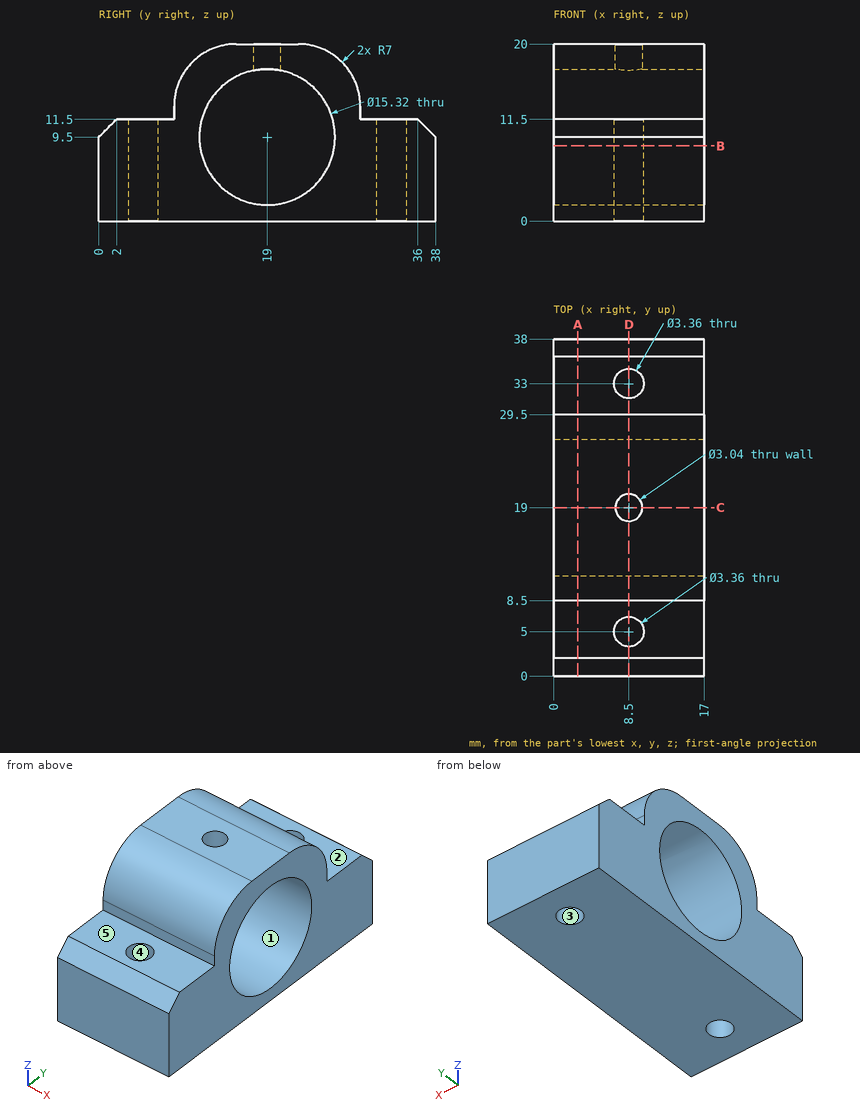
Design review of the part shown in the three views and the two pictorial views. Dimensions are in mm from the part's minimum x, y and z. A direction names the side the tool comes from. Round coordinates to 2 decimals unless told otherwise and drop trailing zeros. Loops run counter-clockwise (first coordinate to the right, second up) from the corner with the lowest first, then second, coordinate; pieces in that order, holes last. Notation, with made-up numbers: M 13.25,-14 L 66.25,-14 A24 ccw 66.25,25 Z; hole C 10.25,24 d11. An arc over 180 degrees is marked long. Write item = value, one per line.
Item 1: Take a section at A-A on x = 2.75. Write out the cut boundary in (y, z).
Return value:
outline = M 0,0 L 38,0 L 38,9.5 L 36,11.5 L 29.5,11.5 L 29.5,13 A7 ccw 22.5,20 L 15.5,20 A7 ccw 8.5,13 L 8.5,11.5 L 2,11.5 L 0,9.5 Z; hole C 19,9.5 d15.32
Item 2: For line 1 (Z direction, x = 13, y = 19); line 2 (X direction, y = 19, z = 17.6); line 3 (X direction, y = 33, z = 8), list the stretches that pass through material, from the lowest coordinate up. Write a range as [from, to].
Return value:
line_1 = [0, 1.84], [17.16, 20]
line_2 = [0, 6.98], [10.02, 17]
line_3 = [0, 6.82], [10.18, 17]
Item 3: Insertion check: P1, Ø2, axis at x = 4.5, z = 11, coming from the -Y side; P2, Ø1.5, axis at y = 21.5, z = 4, coming from the -X side; P3, Ø2, axis at x = 3.5, y = 25, coming from the +Z side; P4, Ø1.2, axis at x = 9.5, z = 12, coming from the +Y side. Each pin has a flat end and moves straight along its axis. Give the tip position at first contact, or say it passes through.
Return value:
P1 = 0.5
P2 = through
P3 = 19.84
P4 = 36.1
Item 4: Machinability: for the marked faces 4 and 5, which of the approach directions +Z, -Z, +X, -X, +Y, -Y give a long, thin tool a straight path to every point of the face, cutting with its end or side? Answer none if there is none.
Return value:
face_4 = +Z, -Z
face_5 = +Z, +X, -X, -Y
Item 5: Take a section at C-C on y = 19. Write out the cut boundary in (x, z).
Return value:
outline = M 0,0 L 17,0 L 17,1.84 L 0,1.84 Z; M 0,17.16 L 6.98,17.16 L 6.98,20 L 0,20 Z; M 10.02,17.16 L 17,17.16 L 17,20 L 10.02,20 Z
Item 6: The part is to be moulded in two halves that separate along Z. For the marked faces 1, 2 and 3, say which applies: released by +Z, released by -Z, zero draft, split by the parting line, or undercut.
Return value:
face_1 = undercut
face_2 = released by +Z
face_3 = zero draft
Item 7: Take a section at D-D on x = 8.5. Write out the cut boundary in (y, z).
Return value:
outline = M 0,0 L 3.32,0 L 3.32,11.5 L 2,11.5 L 0,9.5 Z; M 6.68,0 L 31.32,0 L 31.32,11.5 L 29.5,11.5 L 29.5,13 A7 ccw 22.5,20 L 20.52,20 L 20.52,17.01 A7.66 cw long 17.48,17.01 L 17.48,20 L 15.5,20 A7 ccw 8.5,13 L 8.5,11.5 L 6.68,11.5 Z; M 34.68,0 L 38,0 L 38,9.5 L 36,11.5 L 34.68,11.5 Z
Item 8: Take a section at B-B on z = 8.5. Write out the cut boundary in (x, y), then the cut area to 3 significant figures.
Return value:
outline = M 0,0 L 17,0 L 17,11.41 L 0,11.41 Z; M 0,26.59 L 17,26.59 L 17,38 L 0,38 Z; hole C 8.5,5 d3.36; hole C 8.5,33 d3.36
area = 370 mm2
